Read the model definition and answer for the solid it produces. Units are mm, in the model's axes. A direction names the side the tool comes from. Give positions to 0.01 mm unless a question says otherwise; leave off trailing zeros. Order: outer loops, then holes, each group sorted by start corner. A loop starts at its lowest first (then second) coordinate and runs counter-clockwise, first axis right, second up. Notation, with made-up numbers: (83, 49.25) - (125, 49.25) arc R31 ccw to (125, 76.25) - close; hole circle Ø8 at (45.5, 46.25). An arc over 180 degrees is marked (long way). Write item = value, one per line.
```python
from build123d import *

# Parameters (mm, degrees)
SKETCH_1_W          = 180
SKETCH_1_H          = 50
EXTRUDE_1_DEPTH     = 10
SKETCH_2_W          = 40
SKETCH_2_H          = 50
EXTRUDE_2_DEPTH     = 60
FILLET_1_R          = 25
SKETCH_3_R          = 12.5
CUT_EXTRUDE_2_DEPTH = 135.907375632


with BuildPart() as part:
    # 草图1 → 凸台-拉伸1 (new body)
    with BuildSketch(Plane(origin=(0, 0, 0), x_dir=(1, 0, 0), z_dir=(0, 1, 0))):
        with Locations((90, -25)):
            Rectangle(SKETCH_1_W, SKETCH_1_H)
    extrude(amount=EXTRUDE_1_DEPTH)

    # 草图2 → 凸台-拉伸2 (add)
    with BuildSketch(Plane.XZ):
        with Locations((90, 25)):
            Rectangle(SKETCH_2_W, SKETCH_2_H)
    extrude(amount=EXTRUDE_2_DEPTH)

    # 圆角1
    fillet_1_edges = [part.edges().sort_by_distance(p)[0] for p in [
        (90, -60, 50),
        (90, -60, 0),
    ]]
    fillet(fillet_1_edges, radius=FILLET_1_R - 0.0001)  # a hair under: the kernel refuses the full size

    # 草图3 → 切除-拉伸2 (cut, through all)
    with BuildSketch(Plane(origin=(110, 0, 0), x_dir=(0, 0, -1), z_dir=(1, 0, 0))):
        with Locations((-25, -35)):
            Circle(SKETCH_3_R)
    extrude(amount=-CUT_EXTRUDE_2_DEPTH, mode=Mode.SUBTRACT)


solid = part.part
```
1. Section A-A (z = 17.5) is taken. Determine the outline of the cut face in (x, y), and give its area (3 significant figures).
Recorded:
outline = (0, 0) - (70, 0) - (70, -25) - (110, -25) - (110, 0) - (180, 0) - (180, 10) - (0, 10) - close; (70, -58.85) - (110, -58.85) - (110, -45) - (70, -45) - close
area = 3,350 mm^2
2. Section D-D (z = 46) is taken. Determine the outline of the cut face in (x, y).
Recorded:
outline = (0, 0) - (70, 0) - (70, -48.56) - (110, -48.56) - (110, 0) - (180, 0) - (180, 10) - (0, 10) - close
3. Determine the mould class of faces 1 (the face through (70, -23, 19)), 2 (the face through (90.28, -26.55, 34.21)), 3 (the face through (90.28, -52.482, 7.129)), 4 (the face through (89, -3, 50)) for opening direction Z: +Z half, -Z half, draft (parallel to the pull), parting line (faces both ways), or undercut.
Recorded:
face_1 = draft
face_2 = undercut
face_3 = -Z half
face_4 = +Z half
4. Straight lines are drawn through the part: L1, parallel to Y at x = 90, z = 25; L2, parallel to X at y = -50, z = 23; L3, parallel to Y at x = 111.5, z = 3. For each, find the intervals that lie inside material, in ascending order. Write a range as [from, to].
Recorded:
L1 = [-60, -47.5], [-22.5, 10]
L2 = [70, 110]
L3 = [0, 10]
5. Section C-C (y = -16) is taken. Determine the outline of the cut face in (x, z).
Recorded:
outline = (70, 0) - (110, 0) - (110, 50) - (70, 50) - close
6. For faces 5 (the face through (35, 0, 25)), 6 (the face through (145, 0, 25)), 7 (the face through (89, -3, 0)), determine the directions among +Z, -Z, +X, -X, +Y, -Y from which every point of the face is accessible in a straight line to the end or side of a thin tool.
Recorded:
face_5 = +Z, -Z, -X, -Y
face_6 = +Z, -Z, +X, -Y
face_7 = -Z, +X, -X, +Y, -Y
7. Flat-ended cylindrical pins translate along their axes: pin 1 (4 mm diameter, centred on y = -25.5, z = 12, fed in from +X); pin 2 (1 mm diameter, centred on x = 132, z = 23, fed in from -Y); pin 3 (8 mm diameter, centred on x = 72.5, y = -52, fed in from -Z). Find the tip coordinate at first contact, or state that the pin passes through.
Recorded:
pin_1 = 110
pin_2 = 0
pin_3 = 3.65
